Read the model definition and answer for the solid it produces. Units are mm, in the model's axes. Face numbers are marked on the shaded views. A direction names the side the tool comes from. Round coordinates to 2 decimals unless told otherwise and drop trailing zeros. Order: outer loops, then holes, each group sorted by start corner. A loop starts at its lowest first (then second) coordinate and runs counter-clockwise, first axis right, second up.
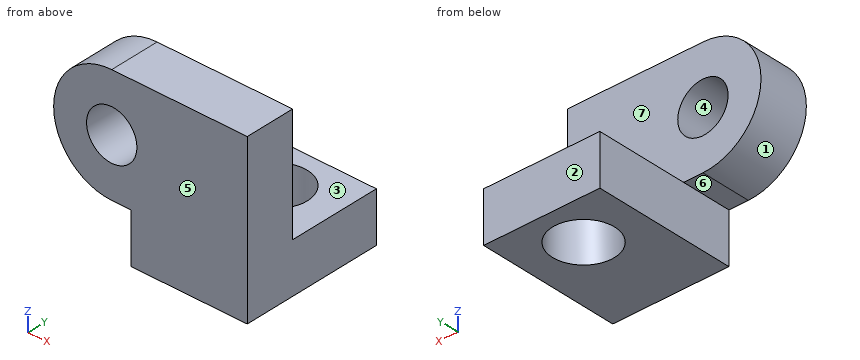
from build123d import *

# Parameters (mm, degrees)
SKETCH1_R           = 6.5
BOSS_EXTRUDE1_DEPTH = 13
SKETCH2_W           = 30
SKETCH2_H           = 13
BOSS_EXTRUDE2_DEPTH = 37
SKETCH3_R           = 8
CUT_EXTRUDE1_DEPTH  = 43


with BuildPart() as part:
    # Sketch1 → Boss-Extrude1 (new body)
    with BuildSketch(Plane(origin=(0, 0, 0), x_dir=(1, 0, 0), z_dir=(0, 1, 0))):
        with BuildLine():
            Line((0, 0), (-35, 0))
            ThreePointArc((-35, 0), (-50, 15), (-35, 30))
            Line((-35, 30), (0, 30))
            Line((0, 30), (0, 0))
        make_face()
        with Locations((-35, 15)):
            Circle(SKETCH1_R, mode=Mode.SUBTRACT)
    extrude(amount=BOSS_EXTRUDE1_DEPTH)

    # Sketch2 → Boss-Extrude2 (add)
    with BuildSketch(Plane(origin=(0, 0, 0), x_dir=(1, 0, 0), z_dir=(0, 1, 0))):
        with Locations((-15, 36.5)):
            Rectangle(SKETCH2_W, SKETCH2_H)
    extrude(amount=BOSS_EXTRUDE2_DEPTH)

    # Sketch3 → Cut-Extrude1 (cut)
    with BuildSketch(Plane.XY):
        with Locations((-15, 25)):
            Circle(SKETCH3_R)
    extrude(amount=-CUT_EXTRUDE1_DEPTH, mode=Mode.SUBTRACT)


solid = part.part
Q1. For the marked faces 5, 6 and 7, determine the directions among +Z, -Z, +X, -X, +Y, -Y from which every point of the face is accessible in a straight line to the end or side of a thin tool.
Outcome:
face 5: +Z, -Z, +X, -X, -Y
face 6: -Z, -X, +Y, -Y
face 7: +Z, +X, -X, +Y
Q2. A cutting plane is placed at B-B, the plane y = 25. Give the vertices of the cut face in (x, z).
Outcome:
outline: (-30, -43) - (-23, -43) - (-23, -30) - (-30, -30) - close; (-7, -43) - (0, -43) - (0, -30) - (-7, -30) - close
Q3. A cutting plane is placed at C-C, the plane z = -33. Give the vertices of the cut face in (x, y), plus the area to 3 significant figures.
Outcome:
outline: (-30, 0) - (0, 0) - (0, 37) - (-30, 37) - close; hole circle Ø16 at (-15, 25)
area: 909 mm2
Q4. Flat-ended cylindrical pins translate along their axes: pin 1 (14.5 mm diameter, centred on y = 22, z = -39, fed in from -X); pin 2 (24 mm diameter, centred on x = -27.5, z = -10, fed in from +Y); pin 3 (5.5 mm diameter, centred on x = -33, y = 6.5, fed in from -Z). Find the tip coordinate at first contact, or state that the pin passes through.
Outcome:
pin 1: stops at x = -30
pin 2: stops at y = 13
pin 3: stops at z = -30
Q5. A cutting plane is placed at A-A, the plane x = -15. Give the vertices of the cut face in (y, z), plus the area to 3 significant figures.
Outcome:
outline: (0, -43) - (17, -43) - (17, -30) - (13, -30) - (13, 0) - (0, 0) - close; (33, -43) - (37, -43) - (37, -30) - (33, -30) - close
area: 663 mm2
Q6. Straight lines are drawn through the part: probe 1 along X at (y, z) = (9, -15); probe 2 along Z at (x, y) = (-35, 4.5); probe 3 along X at (y, z) = (2, -32). For each, find the intervals that lie inside material, in ascending order.
Outcome:
probe 1: x = -50 to -41.5, -28.5 to 0
probe 2: z = -30 to -21.5, -8.5 to 0
probe 3: x = -30 to 0
Q7. For a pull along Z with two mould halves and no side action, classify the marked faces 1, 2, 3 and 4 as released by +Z, released by -Z, zero draft, split by the parting line, or undercut.
Outcome:
face 1: split by the parting line
face 2: zero draft
face 3: released by +Z
face 4: undercut
Q8. A cutting plane is placed at D-D, the plane x = -26. Give the vertices of the cut face in (y, z), plus the area to 3 significant figures.
Outcome:
outline: (0, -43) - (37, -43) - (37, -30) - (13, -30) - (13, 0) - (0, 0) - close
area: 871 mm2
